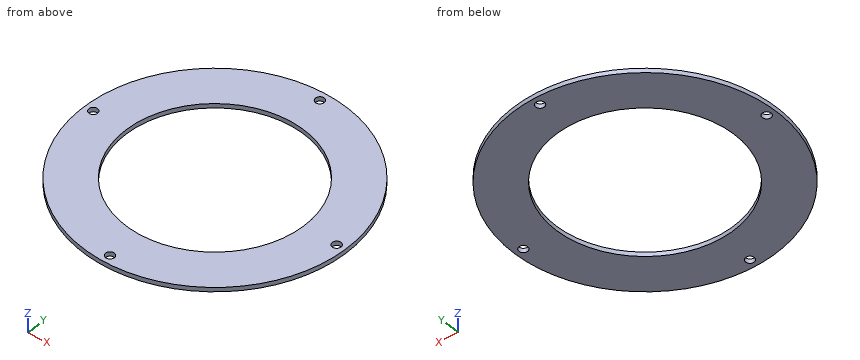
from build123d import *

# Parameters (mm, degrees)
SKETCH_1_R          = 60.5
SKETCH_1_R_2        = 2
SKETCH_1_R_3        = 2.6
SKETCH_1_R_4        = 15.5
EXTRUDE_1_DEPTH     = 2
SKETCH_2_R          = 41
CUT_EXTRUDE_1_DEPTH = 10


with BuildPart() as part:
    # 草图1 → 凸台-拉伸1 (new body)
    with BuildSketch(Plane.XY):
        Circle(SKETCH_1_R)
        with Locations((0, -56.5)):
            Circle(SKETCH_1_R_2, mode=Mode.SUBTRACT)
        with Locations((-56.5, 0)):
            Circle(SKETCH_1_R_2, mode=Mode.SUBTRACT)
        with Locations((0, 56.5)):
            Circle(SKETCH_1_R_2, mode=Mode.SUBTRACT)
        with Locations((56.5, 0)):
            Circle(SKETCH_1_R_2, mode=Mode.SUBTRACT)
        with Locations((0, -23.75)):
            Circle(SKETCH_1_R_3, mode=Mode.SUBTRACT)
        with Locations((-20.56810334, 11.875)):
            Circle(SKETCH_1_R_3, mode=Mode.SUBTRACT)
        with Locations((20.56810334, 11.875)):
            Circle(SKETCH_1_R_3, mode=Mode.SUBTRACT)
        with Locations((19.485571585, -11.25)):
            Circle(SKETCH_1_R_3, mode=Mode.SUBTRACT)
        with Locations((-19.485571585, -11.25)):
            Circle(SKETCH_1_R_3, mode=Mode.SUBTRACT)
        with Locations((0, 22.5)):
            Circle(SKETCH_1_R_3, mode=Mode.SUBTRACT)
        Circle(SKETCH_1_R_4, mode=Mode.SUBTRACT)
    extrude(amount=EXTRUDE_1_DEPTH)

    # 草图2 → 切除-拉伸1 (cut)
    with BuildSketch(Plane.XY.offset(2)):
        Circle(SKETCH_2_R)
    extrude(amount=-CUT_EXTRUDE_1_DEPTH, mode=Mode.SUBTRACT)


solid = part.part
Design review of the part built by this model. Coordinates are the model's own, in mm. Coordinates: 2 decimals unless noted, no trailing zeros. Order: outer loops, then holes, each group sorted by start corner. A loop starts at its lowest first (then second) coordinate and runs counter-clockwise, first axis right, second up. Notation, with made-up numbers: (77, 38) -> (86, 38) arc R17 ccw to (86, 67) -> close; hole circle Ø11 at (18.25, 2). An arc over 180 degrees is marked (long way). One line per item, written item: value.
1) We need section C-C, the plane y = 56.5. Give the boundary of the cut face in (x, z).
Output values:
outline: (-21.63, 0) -> (-2, 0) -> (-2, 2) -> (-21.63, 2) -> close; (2, 0) -> (21.63, 0) -> (21.63, 2) -> (2, 2) -> close
2) To check wall thickness, follow probe 1 along Y at (x, z) = (0, 0.9); probe 2 along X at (y, z) = (-1, 0.65); probe 3 along Y at (x, z) = (44.5, 1.5). State the ranges of each line that lie inside material, in increasing order. Write a range as [from, to].
Output values:
probe 1: y = [-60.5, -58.5], [-54.5, -41], [41, 54.5], [58.5, 60.5]
probe 2: x = [-60.49, -58.23], [-54.77, -40.99], [40.99, 54.77], [58.23, 60.49]
probe 3: y = [-40.99, 40.99]
3) Clearance check with a flat-ended pin moving along its axis: P1, Ø1, axis at y = -38, z = 0.5, coming from the +X side. State where the tip first meets the part, or that it passes through.
Output values:
P1: stops at x = 47.48
4) We need section A-A, the plane y = 0. Give the boundary of the cut face in (x, z).
Output values:
outline: (-60.5, 0) -> (-58.5, 0) -> (-58.5, 2) -> (-60.5, 2) -> close; (-54.5, 0) -> (-41, 0) -> (-41, 2) -> (-54.5, 2) -> close; (41, 0) -> (54.5, 0) -> (54.5, 2) -> (41, 2) -> close; (58.5, 0) -> (60.5, 0) -> (60.5, 2) -> (58.5, 2) -> close
